Geometry: final body of the model. Coordinates: model frame, mm. A direction names the side the tool comes from. Coordinates: 2 decimals unless noted, no trailing zeros. Order: outer loops, then holes, each group sorted by start corner. A loop starts at its lowest first (then second) coordinate and runs counter-clockwise, first axis right, second up. Notation, with made-up numbers: (78.5, 2.5) -> (91.5, 2.5) arc R7 cw to (91.5, 6.5) -> close; hole circle Ø1 at (13, 0.25). An arc over 180 degrees is marked (long way). Answer in a Markdown table with one row per item. Add a question column.
1) Contact query for a flat-ended pin moving along its axis: P1, Ø4, axis at x = 7, y = 16, coming from the -Z side. Output: stop coordinate, or through.
2) Pull-direction query (Y, two-part tool) for faces 1 (the face through (44, 9, 2)), 2 (the face through (-4.14, -9.1, 1.97)), 3 (the face through (22, 26, 0)), 4 (the face through (0, 10, 2)); classes: +Y half, -Y half, draft (parallel to the pull), parting line (faces both ways), or undercut.
3) Set-up query: faces 5 (the face through (22, 19, 2)), 6 (the face through (48.1, -9.14, 1.97)). Return all of +Z, -Z, +X, -X, +Y, -Y with unobstructed straight access to the full face (end or side cutting, diameter ignored); none if empty.
4) Section query D-D on x = 37. Return the cut outline in (y, z), then the cut area to 3 significant figures.
5) Section query C-C on y = 33. Return the cut outline in (x, z), then the cut area to 3 significant figures.
6) Ray query, line 1 (X direction, y = 31.5, z = 3.6); line 2 (Y direction, x = 13, z = 3.3); line 3 (X direction, y = 6.5, z = 3.8). Return the intervals inside material, ascending. Write a range as from..to.
7) Section query B-B on z = 0.75. Return the cut outline in (x, y).
8) Section query A-A on x = 21. Return the cut outline in (y, z).
```python
from build123d import *

# Parameters (mm, degrees)
SKETCH1_W           = 4
SKETCH1_H           = 15
BOSS_EXTRUDE1_DEPTH = 4


with BuildPart() as part:
    # Sketch1 → Boss-Extrude1 (new body)
    with BuildSketch(Plane.XY):
        with BuildLine():
            Line((-2, -10), (46, -10))
            ThreePointArc((46, -10), (48.121320344, -9.121320344), (49, -7))
            Line((49, -7), (49, 46))
            ThreePointArc((49, 46), (48.121320344, 48.121320344), (46, 49))
            Line((46, 49), (-2, 49))
            ThreePointArc((-2, 49), (-4.121320344, 48.121320344), (-5, 46))
            Line((-5, 46), (-5, -7))
            ThreePointArc((-5, -7), (-4.121320344, -9.121320344), (-2, -10))
        make_face()
        with BuildLine():
            Line((3, 0), (41, 0))
            ThreePointArc((41, 0), (43.121320344, 0.878679656), (44, 3))
            Line((44, 3), (44, 16))
            ThreePointArc((44, 16), (43.121320344, 18.121320344), (41, 19))
            Line((41, 19), (3, 19))
            ThreePointArc((3, 19), (0.878679656, 18.121320344), (0, 16))
            Line((0, 16), (0, 3))
            ThreePointArc((0, 3), (0.878679656, 0.878679656), (3, 0))
        make_face(mode=Mode.SUBTRACT)
        with Locations((22, 36.5)):
            Rectangle(SKETCH1_W, SKETCH1_H, mode=Mode.SUBTRACT)
    extrude(amount=BOSS_EXTRUDE1_DEPTH)


solid = part.part
```
Result:
| question | item | result |
|---|---|---|
| 1 | P1 | through |
| 2 | face 1 | undercut |
| 2 | face 2 | -Y half |
| 2 | face 3 | draft |
| 2 | face 4 | undercut |
| 3 | face 5 | +Z, -Z |
| 3 | face 6 | +Z, -Z, +X, -Y |
| 4 | outline | (-10, 0) -> (0, 0) -> (0, 4) -> (-10, 4) -> close; (19, 0) -> (49, 0) -> (49, 4) -> (19, 4) -> close |
| 4 | area | 160 mm2 |
| 5 | outline | (-5, 0) -> (20, 0) -> (20, 4) -> (-5, 4) -> close; (24, 0) -> (49, 0) -> (49, 4) -> (24, 4) -> close |
| 5 | area | 200 mm2 |
| 6 | line 1 | -5..20, 24..49 |
| 6 | line 2 | -10..0, 19..49 |
| 6 | line 3 | -5..0, 44..49 |
| 7 | outline | (-5, -7) arc R3 ccw to (-2, -10) -> (46, -10) arc R3 ccw to (49, -7) -> (49, 46) arc R3 ccw to (46, 49) -> (-2, 49) arc R3 ccw to (-5, 46) -> close; hole (0, 3) arc R3 ccw to (3, 0) -> (41, 0) arc R3 ccw to (44, 3) -> (44, 16) arc R3 ccw to (41, 19) -> (3, 19) arc R3 ccw to (0, 16) -> close; hole (20, 29) -> (24, 29) -> (24, 44) -> (20, 44) -> close |
| 8 | outline | (-10, 0) -> (0, 0) -> (0, 4) -> (-10, 4) -> close; (19, 0) -> (29, 0) -> (29, 4) -> (19, 4) -> close; (44, 0) -> (49, 0) -> (49, 4) -> (44, 4) -> close |
